Could you check a few things on this model? Use its own coordinates, in mm. Face numbers are marked on the shaded views. A direction names the side the tool comes from. Round coordinates to 2 decimals unless told otherwise and drop trailing zeros. Loops run counter-clockwise (first coordinate to the right, second up) from the corner with the lowest first, then second, coordinate; pieces in that order, holes last. Notation, with made-up numbers: (-23, -35) - (8, -35) arc R6 ccw to (8, -31) - close; hole circle Ø10 at (-36.75, 79.25). An arc over 180 degrees is marked (long way). Answer as CSV lines item,"result". Start each with the question number.
1) I'm going to push flat-ended pins straight in: pin 1 Ø6.5 at (y, z) = (20, -13) entering from -X; pin 2 Ø1.8 at (x, y) = (-90.5, 19.5) entering from +Z; pin 3 Ø1.5 at (y, z) = (74, -24.5) entering from -X; pin 4 Ø12 at (y, z) = (72, -17) entering from -X. Where does each tip first touch, or does it pass through?
2) Suppose I cut it at C-C, the plane z = -36. Write out the boundary of the cut face in (x, y).
3) Suppose I cut it at D-D, the plane x = 16. Write out the boundary of the cut face in (y, z).
4) We'd pull the mould along Z, two halves only. Please class the marked faces 1, 2 and 3: pulls with the +Z half, pulls with the -Z half, needs draft (parallel to the pull), parting line crosses it, or undercut.
5) Which directions (+Z, -Z, +X, -X, +Y, -Y) give clear straight access to the entire face, cutting with the end or side of a thin tool? Please do the marked faces 4, 5, 6 and 7.
6) Please list where these lines run through material, in increasing order: line 1 along X through (y, z) = (62.5, -33); line 2 along Y through (x, z) = (13, -56); line 3 along Y through (x, z) = (-74, -38).
7) Suppose I cut it at A-A, the plane x = -70. Write out the boundary of the cut face in (y, z).
8) Suppose I cut it at B-B, the plane y = 31. Write out the boundary of the cut face in (x, z), then the cut area to 3 significant figures.
```python
from build123d import *

# Parameters (mm, degrees)
BOSS_EXTRUDE7_DEPTH      = 72
CUT_EXTRUDE4_DEPTH       = 72
BOSS_EXTRUDE8_DEPTH      = 36
CUT_EXTRUDE10_DEPTH      = 30
SKETCH17_R               = 12
CUT_EXTRUDE11_DEPTH      = 30
CUT_EXTRUDE11_DEPTH_BACK = 1


with BuildPart() as part:
    # Sketch7 → Boss-Extrude7 (new body)
    with BuildSketch(Plane.XY):
        Polygon((-85.777777778, 17.777777778), (-13.777777778, 17.777777778), (-13.777777778, 12.777777778), (59.222222222, 12.777777778), (59.222222222, 37.777777778), (-13.777777778, 37.777777778), (-37.777777778, 37.777777778), (-37.777777778, 97.777777778), (-73.777777778, 97.777777778), (-73.777777778, 73.777777778), (-61.777777778, 73.777777778), (-61.777777778, 47.777777778), (-73.777777778, 47.777777778), (-85.777777778, 47.777777778), align=None)
    extrude(amount=-BOSS_EXTRUDE7_DEPTH)

    # Sketch9 → Cut-Extrude4 (cut)
    with BuildSketch(Plane(origin=(0, 37.777777778, 0), x_dir=(1, 0, 0), z_dir=(0, 1, 0))):
        with BuildLine():
            Line((59.222222222, 24), (9.222222222, 24))
            ThreePointArc((9.222222222, 24), (-2.777777778, 36), (9.222222222, 48))
            Line((9.222222222, 48), (59.222222222, 48))
            Line((59.222222222, 48), (59.222222222, 24))
        make_face()
    extrude(amount=-CUT_EXTRUDE4_DEPTH, mode=Mode.SUBTRACT)

    # Sketch12 → Boss-Extrude8 (add)
    with BuildSketch(Plane.ZY.offset(62)):
        with BuildLine():
            ThreePointArc((-61, 47.777777778), (-36, 34.36090173), (-11, 47.777777778))
            Line((-11, 47.777777778), (0, 47.777777778))
            Line((0, 47.777777778), (0, 23.789694875))
            Line((0, 23.789694875), (-50, 23.789694875))
            Line((-50, 23.789694875), (-50, 17.777777778))
            Line((-50, 17.777777778), (-72, 17.777777778))
            Line((-72, 17.777777778), (-72, 47.777777778))
            Line((-72, 47.777777778), (-61, 47.777777778))
        make_face()
        with BuildLine():
            Line((-72, 73.777777778), (-61, 73.777777778))
            ThreePointArc((-61, 73.777777778), (-36, 87.194653826), (-11, 73.777777778))
            Line((-11, 73.777777778), (0, 73.777777778))
            Line((0, 73.777777778), (0, 97.777777778))
            Line((0, 97.777777778), (-72, 97.777777778))
            Line((-72, 97.777777778), (-72, 73.777777778))
        make_face()
    extrude(amount=BOSS_EXTRUDE8_DEPTH)

    # Sketch13 → Cut-Extrude10 (cut)
    with BuildSketch(Plane.ZY.offset(62)):
        with BuildLine():
            ThreePointArc((-11, 47.777777778), (-36, 34.36090173), (-61, 47.777777778))
            Line((-61, 47.777777778), (-11, 47.777777778))
        make_face()
        with BuildLine():
            ThreePointArc((-61, 73.777777778), (-36, 87.194653826), (-11, 73.777777778))
            Line((-11, 73.777777778), (-28.562094012, 73.777777778))
            Line((-28.562094012, 73.777777778), (-43.437905988, 73.777777778))
            Line((-43.437905988, 73.777777778), (-61, 73.777777778))
        make_face()
    extrude(amount=CUT_EXTRUDE10_DEPTH, mode=Mode.SUBTRACT)

    # Sketch17 → Cut-Extrude11 (cut, two sides)
    with BuildSketch(Plane.ZY.offset(61.777777778)) as cut_extrude11_sk:
        with Locations((-35.93265931, 64.574548991)):
            Circle(SKETCH17_R)
    extrude(amount=CUT_EXTRUDE11_DEPTH, mode=Mode.SUBTRACT)
    extrude(cut_extrude11_sk.sketch, amount=-CUT_EXTRUDE11_DEPTH_BACK, mode=Mode.SUBTRACT)


solid = part.part
```
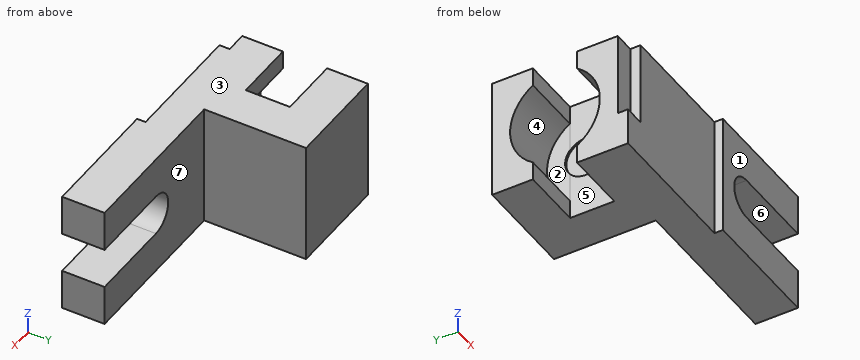
Filled sheet:
1,pin 1,"x = -85.78"
1,pin 2,"z = -50"
1,pin 3,"x = -62"
1,pin 4,"x = -98"
2,outline,"(-98, 23.79) - (-85.78, 23.79) - (-85.78, 17.78) - (-13.78, 17.78) - (-13.78, 12.78) - (-2.78, 12.78) - (-2.78, 37.78) - (-37.78, 37.78) - (-37.78, 97.78) - (-98, 97.78) - (-98, 87.19) - (-62, 87.19) - (-62, 76.57) - (-60.78, 76.57) - (-60.78, 52.57) - (-61.78, 52.57) - (-61.78, 47.78) - (-62, 47.78) - (-62, 34.36) - (-98, 34.36) - close"
3,outline,"(12.78, -72) - (37.78, -72) - (37.78, -48) - (12.78, -48) - close; (12.78, -24) - (37.78, -24) - (37.78, 0) - (12.78, 0) - close"
4,face 1,"needs draft"
4,face 2,"undercut"
4,face 3,"pulls with the +Z half"
5,face 4,"-X"
5,face 5,"+Z, -Z, -X"
5,face 6,"+X, +Y, -Y"
5,face 7,"+Z, -Z, +X, +Y"
6,line 1,"-60.78 to -37.78"
6,line 2,"12.78 to 37.78"
6,line 3,"17.78 to 34.43, 87.13 to 97.78"
7,outline,"(17.78, -72) - (47.78, -72) - (47.78, -61) arc R30 cw to (47.78, -11) - (47.78, 0) - (17.78, 0) - close; (73.78, -72) - (97.78, -72) - (97.78, 0) - (73.78, 0) - (73.78, -11) arc R30 cw to (73.78, -61) - close"
8,outline,"(-98, -72) - (59.22, -72) - (59.22, -48) - (9.22, -48) arc R12 cw to (9.22, -24) - (59.22, -24) - (59.22, 0) - (-98, 0) - close"
8,area,"9,890 mm²"
